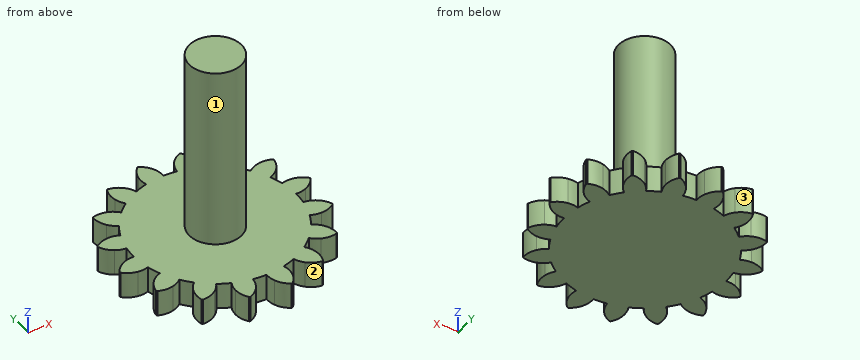
```python
from build123d import *

# Parameters (mm, degrees)
F1_DEPTH = 1.5875
F2_COUNT = 16
F0_R     = 1.5875
F3_DEPTH = 1.5875
F4_DEPTH = 12.7


# Not quite as in the source:
# - a length typed as a fraction of an inch, garbled in the dataset ("3 / 203.2 mm" for 3/8 in), is restored


with BuildPart() as f1:
    # F0 (on Top) → F1 (new body)
    with BuildSketch(Plane.XY):
        with BuildLine():
            ThreePointArc((-1.051103421, 4.8804715195), (-0.4854789746, 4.9694364781), (0.0866333591, 4.9925288117))
            ThreePointArc((0.0866333591, 4.9925288117), (0.0808731678, 5.3155254225), (-7.85e-08, 5.6282865269))
            ThreePointArc((-7.85e-08, 5.6282865269), (-0.2339701384, 6.0238183846), (-0.5826076907, 6.3232166086))
            ThreePointArc((-0.5826076907, 6.3232166086), (-0.6185779348, 6.3208129001), (-0.6543259611, 6.3161529755))
            ThreePointArc((-0.6543259611, 6.3161529755), (-0.9378548446, 5.954491792), (-1.0901647979, 5.5209146738))
            ThreePointArc((-1.0901647979, 5.5209146738), (-1.108467423, 5.1983855986), (-1.051103421, 4.8804715195))
        make_face()
    extrude(amount=F1_DEPTH)


with BuildPart() as f2_1:
    # F2: instance of F1
    add(f1.part.rotate(Axis((-7.85e-08, 0.0402865269, 0), (0, 0, 1)), 1 * 360 / F2_COUNT))


with BuildPart() as f2_2:
    # F2: instance of F1
    add(f1.part.rotate(Axis((-7.85e-08, 0.0402865269, 0), (0, 0, 1)), 2 * 360 / F2_COUNT))


with BuildPart() as f2_3:
    # F2: instance of F1
    add(f1.part.rotate(Axis((-7.85e-08, 0.0402865269, 0), (0, 0, 1)), 3 * 360 / F2_COUNT))


with BuildPart() as f2_4:
    # F2: instance of F1
    add(f1.part.rotate(Axis((-7.85e-08, 0.0402865269, 0), (0, 0, 1)), 4 * 360 / F2_COUNT))


with BuildPart() as f2_5:
    # F2: instance of F1
    add(f1.part.rotate(Axis((-7.85e-08, 0.0402865269, 0), (0, 0, 1)), 5 * 360 / F2_COUNT))


with BuildPart() as f2_6:
    # F2: instance of F1
    add(f1.part.rotate(Axis((-7.85e-08, 0.0402865269, 0), (0, 0, 1)), 6 * 360 / F2_COUNT))


with BuildPart() as f2_7:
    # F2: instance of F1
    add(f1.part.rotate(Axis((-7.85e-08, 0.0402865269, 0), (0, 0, 1)), 7 * 360 / F2_COUNT))


with BuildPart() as f2_8:
    # F2: instance of F1
    add(f1.part.rotate(Axis((-7.85e-08, 0.0402865269, 0), (0, 0, 1)), 8 * 360 / F2_COUNT))


with BuildPart() as f2_9:
    # F2: instance of F1
    add(f1.part.rotate(Axis((-7.85e-08, 0.0402865269, 0), (0, 0, 1)), 9 * 360 / F2_COUNT))


with BuildPart() as f2_10:
    # F2: instance of F1
    add(f1.part.rotate(Axis((-7.85e-08, 0.0402865269, 0), (0, 0, 1)), 10 * 360 / F2_COUNT))


with BuildPart() as f2_11:
    # F2: instance of F1
    add(f1.part.rotate(Axis((-7.85e-08, 0.0402865269, 0), (0, 0, 1)), 11 * 360 / F2_COUNT))


with BuildPart() as f2_12:
    # F2: instance of F1
    add(f1.part.rotate(Axis((-7.85e-08, 0.0402865269, 0), (0, 0, 1)), 12 * 360 / F2_COUNT))


with BuildPart() as f2_13:
    # F2: instance of F1
    add(f1.part.rotate(Axis((-7.85e-08, 0.0402865269, 0), (0, 0, 1)), 13 * 360 / F2_COUNT))


with BuildPart() as f2_14:
    # F2: instance of F1
    add(f1.part.rotate(Axis((-7.85e-08, 0.0402865269, 0), (0, 0, 1)), 14 * 360 / F2_COUNT))


with BuildPart() as f2_15:
    # F2: instance of F1
    add(f1.part.rotate(Axis((-7.85e-08, 0.0402865269, 0), (0, 0, 1)), 15 * 360 / F2_COUNT))


with BuildPart() as f1_1:
    add(f1.part)

    add(f2_1.part)  # F3 merges F2_1

    add(f2_2.part)  # F3 merges F2_2

    add(f2_3.part)  # F3 merges F2_3

    add(f2_4.part)  # F3 merges F2_4

    add(f2_5.part)  # F3 merges F2_5

    add(f2_6.part)  # F3 merges F2_6

    add(f2_7.part)  # F3 merges F2_7

    add(f2_8.part)  # F3 merges F2_8

    add(f2_9.part)  # F3 merges F2_9

    add(f2_10.part)  # F3 merges F2_10

    add(f2_11.part)  # F3 merges F2_11

    add(f2_12.part)  # F3 merges F2_12

    add(f2_13.part)  # F3 merges F2_13

    add(f2_14.part)  # F3 merges F2_14

    add(f2_15.part)  # F3 merges F2_15
    # F0 (on Top) → F3 (join)
    with BuildSketch(Plane.XY):
        with BuildLine():
            ThreePointArc((-1.051103421, 4.8804715195), (-3.1085442832, -3.815768702), (4.9529999215, 0.0402865269))
            ThreePointArc((4.9529999215, 0.0402865269), (3.5327965769, 3.511821748), (0.0866333591, 4.9925288117))
            ThreePointArc((0.0866333591, 4.9925288117), (-0.4854789746, 4.9694364781), (-1.051103421, 4.8804715195))
        make_face()
        Circle(F0_R, mode=Mode.SUBTRACT)
    extrude(amount=F3_DEPTH)

    # F0 (on Top) → F4 (join)
    with BuildSketch(Plane.XY):
        Circle(F0_R)
    extrude(amount=F4_DEPTH)


solid = f1_1.part
```
Could you check a few things on this model? Use its own coordinates, in mm. Face numbers are marked on the shaded views. A direction names the side the tool comes from. Give positions to 0.01 mm unless a question says otherwise; leave off trailing zeros. Order: outer loops, then holes, each group sorted by start corner. A loop starts at its lowest first (then second) coordinate and runs counter-clockwise, first axis right, second up.
Q1. For the marked faces 1, 2 and 3, which set-ups out of +Z, -Z, +X, -X, +Y, -Y let a thin tool reach every point of the face, with its end or its side?
Q2. Suppose I cut it at B-B, the plane z = 9.25. Write out the boundary of the cut face in (x, y) (1 decimal).
Q3. I'm going to push flat-ended pins straight in: P1, Ø3, axis at x = 3, y = 3.5, coming from the -Z side; P2, Ø4, axis at y = 1, z = 10.5, coming from the +X side; P3, Ø1, axis at y = 3.5, z = 6, coming from the -X side; P4, Ø1, axis at x = -0.5, z = 7.5, coming from the -Y side. Where does each tip first touch, or does it pass through?
Q4. Suppose I cut it at A-A, the plane y = -1.25. Write out the boundary of the cut face in (x, z), and give its area (3 significant figures).
Q5. Suppose I cut it at C-C, the plane y = 2.5. Write out the boundary of the cut face in (x, z), and give its area (3 significant figures).
Q6. If I drill on line 1 along Z through (x, y) = (-1.5, 2); line 2 along X through (y, z) = (1, 5.5); line 3 along X through (y, z) = (-0.5, 4.5), over which ranges is the centre line in solid material (lowest first)?
Solution:
1. face 1: +Z
1. face 2: +Z, -Z, -Y
1. face 3: +Z, -Z, +Y
2. outline: circle Ø3.2 at (0, 0)
3. P1: stops at z = 0
3. P2: stops at x = 1.59
3. P3: passes through
3. P4: stops at y = -1.59
4. outline: (-4.78, 0) - (5.73, 0) - (5.73, 1.59) - (0.98, 1.59) - (0.98, 12.7) - (-0.98, 12.7) - (-0.98, 1.59) - (-4.78, 1.59) - close
4. area: 38.4 mm2
5. outline: (-4.3, 0) - (5.41, 0) - (5.41, 1.59) - (-4.3, 1.59) - close
5. area: 15.4 mm2
6. line 1: z = 0 to 1.59
6. line 2: x = -1.23 to 1.23
6. line 3: x = -1.51 to 1.51
